Autodesk Inventor part; units mm, degrees
ref_plane "Work Plane1" through (-38.4302, 0, 40.64) normal (0, -1, 0) x (-1, 0, 0)
ref_plane "Work Plane2" through (-76.8604, 0, 40.64) normal (0, 0, 1) x (1, 0, 0)
ref_plane "YZ Plane" through (0, 0, 0) normal (1, 0, 0) x (0, 1, 0)
ref_plane "Work Plane1" through (-38.4302, 0, 40.64) normal (0, -1, 0) x (-1, 0, 0)
sketch "Sketch1" plane through (-38.4302, 0, 40.64) normal (0, -1, 0) x (-1, 0, 0)
  circle A0 centre (29.6799, 0) radius 1.8288 construction
  circle A1 centre (-29.6799, 0) radius 1.8288 construction
  line L0 (-34.4805, -7.5946) -> (34.4805, -7.5946) construction
  line L1 (34.4805, -7.5946) -> (34.4805, -19.2786) construction
  line L2 (34.4805, -19.2786) -> (-34.4805, -19.2786) construction
  line L3 (-34.4805, -19.2786) -> (-34.4805, -7.5946) construction
  line L4 (34.4805, 7.5946) -> (-34.4805, 7.5946) construction
  line L5 (-34.4805, 7.5946) -> (-34.4805, 19.2786) construction
  line L6 (-34.4805, 19.2786) -> (34.4805, 19.2786) construction
  line L7 (34.4805, 19.2786) -> (34.4805, 7.5946) construction
  line L8 (-38.4302, 27.94) -> (38.4302, 27.94) construction
  line L9 (-38.4302, -27.94) -> (-38.4302, 27.94) construction
  line L10 (38.4302, -27.94) -> (-38.4302, -27.94) construction
  line L11 (38.4302, 27.94) -> (38.4302, -27.94) construction
  circle A2 centre (-29.6799, 0) radius 1.8288
  circle A3 centre (29.6799, 0) radius 1.8288
  circle A4 centre (29.6799, 0) radius 6.35
  circle A5 centre (-29.6799, 0) radius 6.35
  point P0 (-38.4302, 40.64)
  dimension "d0" = 12.7
  dimension "d1" = 12.7
extrude "Extrusion1" add sketch "Sketch1" along normal blind 3.175
ref_plane "Work Plane2" through (-76.8604, 0, 40.64) normal (0, 0, 1) x (1, 0, 0)
sketch "Sketch2" plane through (-76.8604, 0, 40.64) normal (0, 0, 1) x (1, 0, 0)
  line L0 (10.5791, -3.175) -> (6.9215, -3.175) construction
  line L1 (6.9215, 0) -> (10.5791, 0) construction
  line L2 (69.9389, -3.175) -> (66.2813, -3.175) construction
  line L3 (66.2813, 0) -> (69.9389, 0) construction
  line L4 (6.9215, 0) -> (10.5791, 0) construction
  line L5 (8.7503, 0) -> (68.1101, 0) construction
  line L6 (-4.3871, -3.175) -> (85.3512, -3.175) construction
  circle A0 centre (38.4302, -9.525) radius 2.0574
  circle A1 centre (38.4302, -9.525) radius 6.35 construction
  line L7 (38.4302, 0) -> (38.4302, -31.2723) construction
  circle A2 centre (51.1302, -9.525) radius 2.0574
  arc A3 (51.1302, -15.875) -> (57.4802, -9.525) centre (51.1302, -9.525) ccw
  circle A4 centre (25.7302, -9.525) radius 2.0574
  arc A5 (19.3802, -9.525) -> (25.7302, -15.875) centre (25.7302, -9.525) ccw
  line L8 (25.7302, -15.875) -> (51.1302, -15.875)
  line L9 (19.3802, -3.175) -> (57.4802, -3.175)
  line L10 (19.3802, -9.525) -> (19.3802, -3.175)
  line L11 (57.4802, -9.525) -> (57.4802, -3.175)
  point P0 (76.8604, 0)
  point P1 (25.7302, -3.175)
  point P2 (51.1302, -3.175)
  dimension "d4" = 3.175
  dimension "d5" = 4.1148
  dimension "d6" = 12.7
  dimension "d7" = 4.1148
  dimension "d8" = 12.7
extrude "Extrusion2" add sketch "Sketch2" along normal mid plane 4.7625
sketch "Sketch3" plane through (-68.1101, 0, 40.64) normal (0, 1, 0) x (1, 0, 0)
  circle A0 centre (0, 0) radius 6.35 construction
  circle A1 centre (59.3598, 0) radius 6.35 construction
  line L0 (10.6299, 2.3813) -> (48.7299, 2.3813) construction
  line L1 (48.7299, -2.3812) -> (10.6299, -2.3812) construction
  line L2 (5.8866, 2.3813) -> (53.4732, 2.3813)
  line L3 (5.8866, -2.3812) -> (53.4732, -2.3812)
  circle A2 centre (0, 0) radius 1.8288 construction
  arc A3 (5.8866, -2.3812) -> (5.8866, 2.3813) centre (0, 0) ccw
  circle A4 centre (59.3598, 0) radius 1.8288 construction
  arc A5 (53.4732, 2.3813) -> (53.4732, -2.3812) centre (59.3598, 0) ccw
  point P0 (68.1101, 40.64)
extrude "Extrusion3" add sketch "Sketch3" against normal up to surface (3.175 mm away)
fillet "Fillet1" radius 3.175 2 edges at (-19.3802, -3.175, 40.64) (-57.4802, -3.175, 40.64)
properties part number "ChassisPrototypeA3"
The model under review builds one solid part; all positions refer to its coordinate system, in mm. A direction names the side the tool comes from. Give positions to 0.01 mm unless a question says otherwise; leave off trailing zeros. Write each loop counter-clockwise with the first axis right and the second up, starting at its lowest first coordinate (ties: lowest second). Pieces come first, ordered by that corner, then holes. Notation, with made-up numbers: M -38,13.25 L 17,13.25 A16 ccw 17,38.25 Z; hole C 14.25,51.25 d3. An arc over 180 degrees is marked long. One line per question, with ' | ' between items. Start each with the question number.
Item 1: Draft analysis for pull direction Z (two halves, no side actions). For faces 1 (the cylindrical face through (-2.405, -1.565, 40.885)), 2 (the cylindrical face through (-10.44, -1.57, 39.94)), 3 (the cylindrical face through (-18.425, -4.08, 40.673)), state which applies: released by +Z, released by -Z, zero draft, split by the parting line, or undercut.
Item 2: We need section B-B on z = 44. Write out the cut boundary in (x, y) (3 decimals), plus the area to 3 significant figures.
Item 3: We need section A-A on z = 40.64. Give the number of separate pieces and of enclosed holes in the cut face, plus the area to 3 significant figures.
Item 4: For pin 1 (3 mm diameter, centred on x = -8.75, z = 40.64, fed in from +Y); pin 2 (1 mm diameter, centred on x = -36, y = -1.5, fed in from -Z); pin 3 (2 mm diameter, centred on x = -61.5, z = 39.5, fed in from +Y); pin 4 (6.5 mm diameter, centred on x = -34.5, y = -9, fed in from +Z), all flat-tipped, find the tip position at first contact; note any pin that passes through.
Item 5: For faces 4 (the flat face through (-11, -3.175, 41)), 5 (the flat face through (-57.48, -8, 41)), 6 (the cylindrical face through (-74.455, -1.565, 40.395)), list the 3-axis set-ups (+Z, -Z, +X, -X, +Y, -Y) from which the entire face can be reached by the end or side of a thin tool; tool diameter is ignored.
Item 6: We need section D-D on y = -10.75. Write out the cut boundary in (x, z), plus the area to 3 significant figures.
Item 7: Wall thickness on line 1 (X direction, y = -1.9, z = 40.64); line 2 (X direction, y = -10.25, z = 41.75); line 3 (Z direction, x = -58.5, y = -2.75): over which ranges is each line inside the solid? List them lowest first. Write a range as from..to.
Item 8: We need section C-C on y = -2.5. Write out the cut boundary in (x, z).
Results found:
1) face 1: split by the parting line | face 2: undercut | face 3: zero draft
2) outline: M -73.498,-3.175 L -62.722,-3.175 L -62.722,0 L -73.498,0 Z; M -14.139,-3.175 L -3.362,-3.175 L -3.362,0 L -14.139,0 Z | area: 68.4 mm2
3) separate pieces: 3 | enclosed holes: 3 | area: 637 mm2
4) pin 1: passes through | pin 2: stops at z = 38.26 | pin 3: stops at y = 0 | pin 4: stops at z = 43.02
5) face 4: +Z, -Z, +X, -Y | face 5: +Z, -Z, -X, -Y | face 6: +Y, -Y
6) outline: M -57.36,38.26 L -52.78,38.26 L -52.78,43.02 L -57.36,43.02 Z; M -49.48,38.26 L -40.08,38.26 L -40.08,43.02 L -49.48,43.02 Z; M -36.78,38.26 L -27.38,38.26 L -27.38,43.02 L -36.78,43.02 Z; M -24.08,38.26 L -19.5,38.26 L -19.5,43.02 L -24.08,43.02 Z | area: 133 mm2
7) line 1: x = -74.46..-69.94, -66.28..-10.58, -6.92..-2.4 | line 2: x = -57.44..-53.06, -49.2..-40.36, -36.5..-27.66, -23.8..-19.42 | line 3: z = 38.26..43.02
8) outline: M -62.22,38.26 L -14.64,38.26 A6.35 ccw long -14.64,43.02 L -62.22,43.02 A6.35 ccw long Z; hole C -68.11,40.64 d3.66; hole C -8.75,40.64 d3.66
